```python
from build123d import *

# Parameters (mm, degrees)
SZKIC1_W                    = 80
SZKIC1_H                    = 130
DODANIE_WYCI_GNI_CIE1_DEPTH = 5
ZAOKR_GLENIE1_R             = 10
SZKIC2_W                    = 5
SZKIC2_H                    = 20
DODANIE_WYCI_GNI_CIE2_DEPTH = 18
ZAOKR_GLENIE2_R             = 10
SZKIC3_R                    = 2.5
WYTNIJ_WYCI_GNI_CIE1_DEPTH  = 100


with BuildPart() as part:
    # Szkic1 → Dodanie-wyciągnięcie1 (new body)
    with BuildSketch(Plane(origin=(0, 0, 0), x_dir=(1, 0, 0), z_dir=(0, 1, 0))):
        Rectangle(SZKIC1_W, SZKIC1_H)
    extrude(amount=DODANIE_WYCI_GNI_CIE1_DEPTH)

    # Zaokrąglenie1
    zaokr_glenie1_edges = [part.edges().sort_by_distance(p)[0] for p in [
        (40, 2.5, -65),
        (40, 2.5, 65),
        (-40, 2.5, 65),
        (-40, 2.5, -65),
    ]]
    fillet(zaokr_glenie1_edges, radius=ZAOKR_GLENIE1_R)

    # Szkic2 → Dodanie-wyciągnięcie2 (add)
    with BuildSketch(Plane(origin=(0, 5, 0), x_dir=(1, 0, 0), z_dir=(0, 1, 0))):
        with Locations((-22.5, 25)):
            Rectangle(SZKIC2_W, SZKIC2_H)
        with Locations((22.5, 25)):
            Rectangle(SZKIC2_W, SZKIC2_H)
    extrude(amount=DODANIE_WYCI_GNI_CIE2_DEPTH)

    # Zaokrąglenie2
    zaokr_glenie2_edges = [part.edges().sort_by_distance(p)[0] for p in [
        (22.5, 23, -15),
        (22.5, 23, -35),
        (-22.5, 23, -15),
        (-22.5, 23, -35),
    ]]
    fillet(zaokr_glenie2_edges, radius=ZAOKR_GLENIE2_R - 0.0001)  # a hair under: the kernel refuses the full size

    # Szkic3 → Wytnij-wyciągnięcie1 (cut)
    with BuildSketch(Plane.ZY.offset(25)):
        with Locations((-25, 13)):
            Circle(SZKIC3_R)
    extrude(amount=-WYTNIJ_WYCI_GNI_CIE1_DEPTH, mode=Mode.SUBTRACT)


solid = part.part
```
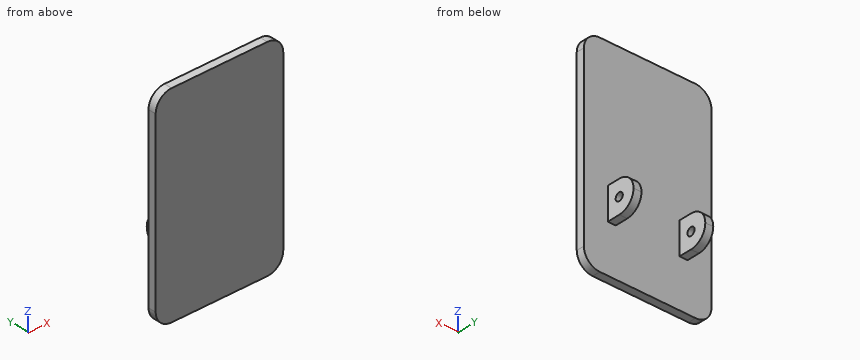
The model under review builds one solid part; all positions refer to its coordinate system, in mm. Round coordinates to 2 decimals unless told otherwise and drop trailing zeros. Loops run counter-clockwise (first coordinate to the right, second up) from the corner with the lowest first, then second, coordinate; pieces in that order, holes last. Notation, with made-up numbers: (-27.5, 66.5) - (-18.5, 66.5) arc R24 ccw to (-18.5, 104.5) - close; hole circle Ø8 at (-31.5, 8.25). An arc over 180 degrees is marked (long way). Use a Markdown table: item, result. Add a question column.
Q1. Add section A-A (y = 17.75). State the section outline as (x, z) points.
Q2. For probe 1 along Y at (x, z) = (21.45, -25); probe 2 along Y at (x, z) = (-37, -33); probe 3 along Z at (x, y) = (-24, 6), list the stretches that pass through material, from the lowest coordinate up.
Q3. Add section C-C (z = -11). State the section outline as (x, y) points, plus the area to 3 significant figures.
Q4. Add section B-B (x = 2.5). State the section outline as (y, z) points, plus the area to 3 significant figures.
Q5. Insertion check: pin 1 Ø4 at (x, y) = (22.5, 10.5) entering from +Z; pin 2 Ø3 at (x, y) = (-25, 16.5) entering from -Z; pin 3 Ø5.5 at (x, y) = (22.5, 8.5) entering from -Z; pin 4 Ø4 at (y, z) = (13, -25) entering from -X. Each pin has a flat end and moves straight along its axis. Give the tip position at first contact, or say it passes through.
Worked answers:
| question | item | result |
|---|---|---|
| 1 | outline | (-25, -33.8) - (-20, -33.8) - (-20, -16.2) - (-25, -16.2) - close; (20, -33.8) - (25, -33.8) - (25, -16.2) - (20, -16.2) - close |
| 2 | probe 1 | 0 to 10.5, 15.5 to 23 |
| 2 | probe 2 | 0 to 5 |
| 2 | probe 3 | -35 to -15 |
| 3 | outline | (-40, 0) - (40, 0) - (40, 5) - (-40, 5) - close |
| 3 | area | 400 mm² |
| 4 | outline | (0, -65) - (5, -65) - (5, 65) - (0, 65) - close |
| 4 | area | 650 mm² |
| 5 | pin 1 | z = -15 |
| 5 | pin 2 | z = -34.8 |
| 5 | pin 3 | z = -35 |
| 5 | pin 4 | through |
